Could you check a few things on this drawing? It's one solid part, dimensions in mm from its lowest x, y, z. A direction names the side the tool comes from. Round coordinates to 2 decimals unless told otherwise and drop trailing zeros. Loops run counter-clockwise (first coordinate to the right, second up) from the corner with the lowest first, then second, coordinate; pieces in that order, holes last. Notation, with made-up numbers: M 39.25,22 L 52.25,22 A18 ccw 52.25,34 Z; hole C -20,82 d7. An arc over 180 degrees is marked long. Return JSON: item names as keys, results as strings.
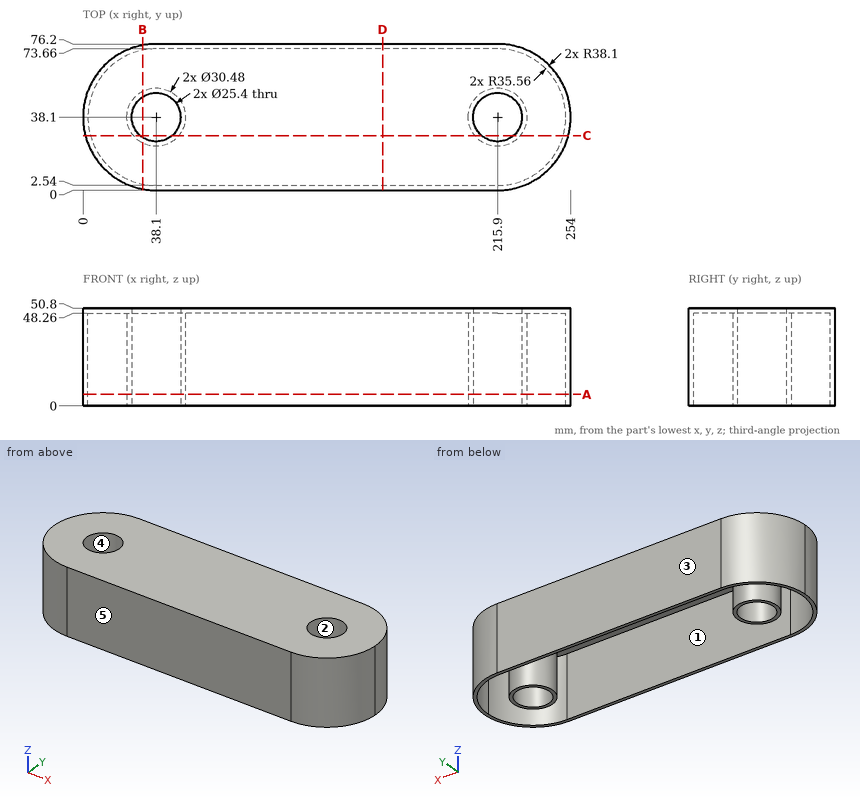
Q1. Suppose I cut it at D-D, the plane x = 156. Please give me the cut outline in (y, z), plus the area to 3 significant figures.
Results:
{"outline": "M 0,0 L 2.54,0 L 2.54,48.26 L 73.66,48.26 L 73.66,0 L 76.2,0 L 76.2,50.8 L 0,50.8 Z", "area": "439 mm2"}
Q2. Thinking about a two-plate mould opening in Y: for the marked faces 3, 4 and 5, which applies, pulls with the +Y half, pulls with the -Y half, needs draft (parallel to the pull), parting line crosses it, or undercut?
Results:
{"face 3": "pulls with the +Y half", "face 4": "undercut", "face 5": "pulls with the -Y half"}
Q3. On a 3-axis mill with a long thin cutter (end or side, diameter ignored), from which of +Z, -Z, +X, -X, +Y, -Y can I reach the whole of each face in a straight line? I mean the marked faces 1 and 2. Say none if no direction works.
Results:
{"face 1": "-Z", "face 2": "+Z, -Z"}
Q4. Suppose I cut it at B-B, the plane x = 31. Please give me the cut outline in (y, z).
Results:
{"outline": "M 0.67,0 L 3.26,0 L 3.26,48.26 L 24.61,48.26 L 24.61,0 L 27.57,0 L 27.57,50.8 L 0.67,50.8 Z; M 48.63,0 L 51.59,0 L 51.59,48.26 L 72.94,48.26 L 72.94,0 L 75.53,0 L 75.53,50.8 L 48.63,50.8 Z"}
Q5. If I drill on line 1 along Y through (x, z) = (215.9, 32); line 2 along Y through (x, z) = (171.5, 12); line 3 along X through (y, z) = (46.5, 36), over which ranges is the centre line in solid material (lowest first)?
Results:
{"line 1": "y = 0 to 2.54, 22.86 to 25.4, 50.8 to 53.34, 73.66 to 76.2", "line 2": "y = 0 to 2.54, 73.66 to 76.2", "line 3": "x = 0.94 to 3.55, 25.38 to 28.57, 47.63 to 50.82, 203.18 to 206.37, 225.43 to 228.62, 250.45 to 253.06"}
Q6. I'm going to push flat-ended pins straight in: pin 1 Ø6 at (y, z) = (24.5, 41.5) entering from +X; pin 2 Ø8 at (y, z) = (21, 13) entering from -X; pin 3 Ø21.5 at (x, y) = (148, 26.5) entering from -Z. Where does each tip first touch, or does it pass through?
Results:
{"pin 1": "stops at x = 252.5", "pin 2": "stops at x = 2.32", "pin 3": "stops at z = 48.26"}
Q7. Suppose I cut it at A-A, the plane z = 6. Please give me the cut outline in (x, y), plus the area to 3 significant figures.
Results:
{"outline": "M 0,38.1 A38.1 ccw 38.1,0 L 215.9,0 A38.1 ccw 254,38.1 A38.1 ccw 215.9,76.2 L 38.1,76.2 A38.1 ccw Z; C 38.1,38.1 d30.48; C 215.9,38.1 d30.48; hole M 2.54,38.1 A35.56 ccw 38.1,2.54 L 215.9,2.54 A35.56 ccw 251.46,38.1 A35.56 ccw 215.9,73.66 L 38.1,73.66 A35.56 ccw Z; hole C 38.1,38.1 d25.4; hole C 215.9,38.1 d25.4", "area": "1,940 mm2"}
Q8. Suppose I cut it at C-C, the plane y = 28.5. Please give me the cut outline in (x, z).
Results:
{"outline": "M 1.23,0 L 3.86,0 L 3.86,48.26 L 26.26,48.26 L 26.26,0 L 29.79,0 L 29.79,50.8 L 1.23,50.8 Z; M 46.41,0 L 49.94,0 L 49.94,48.26 L 204.06,48.26 L 204.06,0 L 207.59,0 L 207.59,50.8 L 46.41,50.8 Z; M 224.21,0 L 227.74,0 L 227.74,48.26 L 250.14,48.26 L 250.14,0 L 252.77,0 L 252.77,50.8 L 224.21,50.8 Z"}
